```python
from build123d import *

# Parameters (mm, degrees)
SKETCH1_W           = 25
SKETCH1_H           = 50
SKETCH1_R           = 3.375
BOSS_EXTRUDE1_DEPTH = 3
SKETCH2_W           = 50
SKETCH2_H           = 3
BOSS_EXTRUDE2_DEPTH = 8
SKETCH3_W           = 8
SKETCH3_H           = 50
BOSS_EXTRUDE3_DEPTH = 42
SKETCH4_R           = 2.65
CUT_EXTRUDE1_DEPTH  = 3.3
SKETCH5_R           = 5.802370205
CUT_EXTRUDE2_DEPTH  = 9
FILLET2_R           = 1
SKETCH6_R           = 12.7
BOSS_EXTRUDE4_DEPTH = 2
FILLET4_R           = 1
SKETCH8_R           = 1.589780168
SKETCH8_R_2         = 1.777428262
CUT_EXTRUDE3_DEPTH  = 10
SKETCH9_W           = 8
SKETCH9_H           = 42
CUT_EXTRUDE4_DEPTH  = 68.79439129


with BuildPart() as part:
    # Sketch1 → Boss-Extrude1 (new body)
    with BuildSketch(Plane(origin=(0, 0, 0), x_dir=(1, 0, 0), z_dir=(0, 1, 0))):
        with Locations((2.276951673, 11.384758364)):
            Rectangle(SKETCH1_W, SKETCH1_H)
        with Locations(Location((1.276951673, 11.384758364, 0), (0, 0, 270))):
            Circle(SKETCH1_R, mode=Mode.SUBTRACT)
    extrude(amount=BOSS_EXTRUDE1_DEPTH)

    # Sketch2 → Boss-Extrude2 (add)
    with BuildSketch(Plane.ZY.offset(10.223048327)):
        with Locations((-11.384758364, 1.5)):
            Rectangle(SKETCH2_W, SKETCH2_H)
    extrude(amount=BOSS_EXTRUDE2_DEPTH)

    # Sketch3 → Boss-Extrude3 (add)
    with BuildSketch(Plane.XZ):
        with Locations((-14.223048327, -11.384758364)):
            Rectangle(SKETCH3_W, SKETCH3_H)
    extrude(amount=BOSS_EXTRUDE3_DEPTH)

    # Sketch4 → Cut-Extrude1 (cut)
    with BuildSketch(Plane(origin=(0, 3, 0), x_dir=(1, 0, 0), z_dir=(0, 1, 0))):
        with Locations(Location((-14.223048327, 32.384758364, 0), (0, 0, 270))):
            Circle(SKETCH4_R)
        with Locations(Location((-14.223048327, -9.615241636, 0), (0, 0, 270))):
            Circle(SKETCH4_R)
    cut_extrude1 = extrude(amount=-CUT_EXTRUDE1_DEPTH, mode=Mode.SUBTRACT)

    # Mirror1: Cut-Extrude1 across plane
    add(cut_extrude1.mirror(Plane.ZX.offset(-19.5)), mode=Mode.SUBTRACT)

    # Sketch5 → Cut-Extrude2 (cut)
    with BuildSketch(Plane.ZY.offset(18.223048327)):
        with Locations((-11.836279124, -21)):
            Circle(SKETCH5_R)
    extrude(amount=-CUT_EXTRUDE2_DEPTH, mode=Mode.SUBTRACT)

    # Fillet2
    fillet2_edges = [part.edges().sort_by_distance(p)[0] for p in [
        (-10.223048327, -21, -17.638649329),
    ]]
    fillet(fillet2_edges, radius=FILLET2_R)

    # Mirror2: Cut-Extrude1 across plane
    add(cut_extrude1.mirror(Plane.ZY.offset(1.723048327)), mode=Mode.SUBTRACT)

    # Sketch6 → Boss-Extrude4 (add)
    with BuildSketch(Plane(origin=(0, 3, 0), x_dir=(1, 0, 0), z_dir=(0, 1, 0))):
        with BuildLine():
            Line((14.776951673, 5.567542535), (14.776951673, 17.201974193))
            ThreePointArc((14.776951673, 17.201974193), (-13.423048327, 11.384758364), (14.776951673, 5.567542535))
        make_face()
        with Locations(Location((1.276951673, 11.384758364, 0), (0, 0, 270))):
            Circle(SKETCH6_R, mode=Mode.SUBTRACT)
    extrude(amount=BOSS_EXTRUDE4_DEPTH)

    # Fillet4
    # the kernel refuses this fillet: 1 mm, written as the material it takes off along each edge
    with BuildSketch(Plane(origin=(14.776951673, 5, -3.067542535), x_dir=(0, -1, 0), z_dir=(0, 0, -1))) as fillet4_piece_1:
        with BuildLine():
            CenterArc((FILLET4_R, FILLET4_R), FILLET4_R, 180, 90)
            Line((0, FILLET4_R), (0, 0))
            Line((0, 0), (FILLET4_R, 0))
        make_face()
    extrude(amount=16.634431658, mode=Mode.SUBTRACT)

    # Sketch8 → Cut-Extrude3 (cut)
    with BuildSketch(Plane(origin=(0, 3, 0), x_dir=(1, 0, 0), z_dir=(0, 1, 0))):
        with Locations(Location((1.276951673, 19.884758364, 0), (0, 0, 270))):
            Circle(SKETCH8_R)
        with Locations(Location((1.276951673, 2.884758364, 0), (0, 0, 270))):
            Circle(SKETCH8_R_2)
    extrude(amount=-CUT_EXTRUDE3_DEPTH, mode=Mode.SUBTRACT)

    # Sketch9 → Cut-Extrude4 (cut, through all)
    with BuildSketch(Plane.XY.offset(13.615241636)):
        with Locations((-14.223048327, -21)):
            Rectangle(SKETCH9_W, SKETCH9_H)
    extrude(amount=-CUT_EXTRUDE4_DEPTH, mode=Mode.SUBTRACT)


solid = part.part
```
Model file for the job. Use its own axes, mm. A direction names the side the tool comes from. Round coordinates to 2 decimals unless told otherwise and drop trailing zeros. Loops run counter-clockwise (first coordinate to the right, second up) from the corner with the lowest first, then second, coordinate; pieces in that order, holes last. Notation, with made-up numbers: M 40.5,-36.5 L 81.5,-36.5 A8 cw 81.5,-27.5 Z; hole C 36.25,45 d10. An arc over 180 degrees is marked long. Put each result on its own line as item: value. Start each with the question number.
Item 1: Cut at C-C (y = 1.3). List the corners of the cut face in (x, z) (3 decimals), then the cut area to 3 significant figures.
Item 2: 3-axis set-ups, long thin cutter, end or side, ignore diameter. For faces 1 (the face through (-6, 0, -11)), 2 (the face through (5.09, 3.99, 0.73)): which of +Z, -Z, +X, -X, +Y, -Y reach the whole face in a straight line?
Item 3: Cut at B-B (x = 4). List the corners of the cut face in (y, z).
Item 4: Drop a flat-ended pin along its axis: P1, Ø15, axis at x = 1.28, z = -11.38, coming from the +Y side. Give the stop position or say it passes through.
Item 5: Mould opens along Z. For faces 3 (the face through (-2, 2, 13.615)), 4 (the face through (-11, 5, -16)), 5 (the face through (1.754, 1.521, -18.368)) say: released by +Z, released by -Z, zero draft, split by the parting line, or undercut.
Item 6: Drill centre lines: line 1 along Z through (x, y) = (0, 2.3); line 2 along Z through (x, y) = (-14.5, 2.9); line 3 along Z through (x, y) = (12, 2.1). Where is each one in solid material? Low to high.
Item 7: Cut at A-A (z = 8.5). List the corners of the cut face in (x, y), then the cut area to 3 significant figures.
Item 8: Cut at D-D (x = -9.5). List the corners of the cut face in (y, z).
Answer block:
1. outline: M -18.223,-36.385 L 14.777,-36.385 L 14.777,13.615 L -18.223,13.615 Z; hole C -14.223,-32.385 d5.3; hole C -14.223,9.615 d5.3; hole C 1.277,-11.385 d6.75; hole C 1.277,-2.885 d3.555; hole C 1.277,-19.885 d3.18; hole C 10.777,-32.385 d5.3; hole C 10.777,9.615 d5.3
1. area: 1,510 mm2
2. face 1: +Z, -Z, +X, -X, -Y
2. face 2: +Y
3. outline: M 0,-36.38 L 3,-36.38 L 3,-25.83 L 5,-25.83 L 5,-23.79 L 3,-23.79 L 3,-13.38 L 0,-13.38 Z; M 0,-9.39 L 3,-9.39 L 3,1.02 L 5,1.02 L 5,3.06 L 3,3.06 L 3,13.62 L 0,13.62 Z
4. P1: y = 3
5. face 3: released by +Z
5. face 4: zero draft
5. face 5: undercut
6. line 1: -36.38 to -20.83, -18.94 to -14.51, -8.26 to -4.12, -1.65 to 13.62
6. line 2: -36.38 to -35.02, -29.75 to 6.98, 12.25 to 13.62
6. line 3: -36.38 to -34.74, -30.03 to 7.26, 11.97 to 13.62
7. outline: M -18.22,0 L -16.63,0 L -16.63,3 L -18.22,3 Z; M -11.82,0 L 8.37,0 L 8.37,3 L -11.82,3 Z; M 13.18,0 L 14.78,0 L 14.78,3 L 13.18,3 Z
7. area: 70.2 mm2
8. outline: M 0,-36.38 L 3,-36.38 L 3,-21.38 L 5,-21.38 L 5,-18.1 L 3,-18.1 L 3,-4.67 L 5,-4.67 L 5,-1.39 L 3,-1.39 L 3,13.62 L 0,13.62 Z
